Source: CAD feature listing. Evaluate the final solid. Frame: model axes, mm. Face numbers are marked on the shaded views. A direction names the side the tool comes from. Give positions to 0.01 mm unless a question says otherwise; leave off trailing zeros. Order: outer loops, then holes, each group sorted by start corner. A loop starts at its lowest first (then second) coordinate and runs counter-clockwise, first axis right, second up. Notation, with made-up numbers: M -2.5,-20.5 L 4.5,-20.5 A22 ccw 4.5,12.5 Z; hole C 2.5,0.25 d7. An arc over 180 degrees is marked long. Answer as a JSON object with one key per item and string values. Group by question number.
1. Pin query (flat end, axial travel): P1, Ø4, axis at x = -46, y = 69, coming from the -Z side; P2, Ø8, axis at x = -45, z = 15, coming from the +Y side; P3, Ø5, axis at y = 58, z = 25, coming from the +X side; P4, Ø1, axis at y = 45, z = 5, coming from the -X side. Return the tip coordinate at first contact, or that it passes through.
2. Set-up query: the marked faces 1 and 2. Return all of +Z, -Z, +X, -X, +Y, -Y with unobstructed straight access to the full face (end or side cutting, diameter ignored); none if empty.
3. Section query B-B (x = -43.75). Output: boundary loops of the cut face in (y, z), plus the area to 3 significant figures.
4. Material intervals for L1, parallel to X at y = 68, z = 29; L2, parallel to Z at x = -42.5, y = 53.5; L3, parallel to Y at x = -52.5, z = 26, sorted ascending. Write a range as [from, to].
5. Section query D-D (y = 65.5). Output: boundary loops of the cut face in (x, z).
6. Section query A-A (z = 27). Output: boundary loops of the cut face in (x, y), plus the area to 3 significant figures.
7. Section query C-C (x = -41.25). Output: boundary loops of the cut face in (y, z).
from build123d import *

# Parameters (mm, degrees)
BOSS_EXTRUDE1_DEPTH = 31.75
SKETCH19_W          = 15.860402013
SKETCH19_H          = 31.75
BOSS_EXTRUDE7_DEPTH = 2
SKETCH23_W          = 15.860402013
SKETCH23_H          = 4
BOSS_EXTRUDE8_DEPTH = 25
SKETCH24_R          = 1.27
CUT_EXTRUDE1_DEPTH  = 5


with BuildPart() as part:
    # Sketch2 → Boss-Extrude1 (new body)
    with BuildSketch(Plane.XY):
        with BuildLine():
            Line((-50.375618534, 45.609862895), (-50.351188886, 46.309436474))
            ThreePointArc((-50.351188886, 46.309436474), (-50.565618587, 46.88295476), (-51.12278195, 47.136868733))
            Line((-51.12278195, 47.136868733), (-55.780902554, 47.299533889))
            Line((-55.780902554, 47.299533889), (-47.850701548, 47.299533889))
            Line((-47.850701548, 47.299533889), (-47.850701548, 40.900752235))
            Line((-47.850701548, 40.900752235), (-48.952946324, 40.900752235))
            ThreePointArc((-48.952946324, 40.900752235), (-50.100996621, 41.129113637), (-51.074266668, 41.779431891))
            Line((-51.074266668, 41.779431891), (-53.375146928, 44.080312152))
            ThreePointArc((-53.375146928, 44.080312152), (-53.536830204, 44.931922499), (-52.803734096, 45.394471696))
            Line((-52.803734096, 45.394471696), (-50.685905631, 45.320515496))
            ThreePointArc((-50.685905631, 45.320515496), (-50.470836274, 45.400926634), (-50.375618534, 45.609862895))
        make_face()
    boss_extrude1 = extrude(amount=BOSS_EXTRUDE1_DEPTH)

    # Mirror2: Boss-Extrude1 across plane
    add(boss_extrude1.mirror(Plane(origin=(-47.850701548, 40.900752235, 31.75), x_dir=(0, 0, 1), z_dir=(-1, 0, 0))))

    # Sketch19 → Boss-Extrude7 (add)
    with BuildSketch(Plane(origin=(0, 47.299533889, 0), x_dir=(1, 0, 0), z_dir=(0, 1, 0))):
        with Locations((-47.850701548, -15.875)):
            Rectangle(SKETCH19_W, SKETCH19_H)
    extrude(amount=BOSS_EXTRUDE7_DEPTH)

    # Sketch23 → Boss-Extrude8 (add)
    with BuildSketch(Plane(origin=(0, 49.299533889, 0), x_dir=(1, 0, 0), z_dir=(0, 1, 0))):
        with Locations((-47.850701548, -29.75)):
            Rectangle(SKETCH23_W, SKETCH23_H)
    extrude(amount=BOSS_EXTRUDE8_DEPTH)

    # Sketch24 → Cut-Extrude1 (cut, through all)
    with BuildSketch(Plane(origin=(0, 0, 27.75), x_dir=(-1, 0, 0), z_dir=(0, 0, -1))):
        with Locations((47.850701548, 67.949533889)):
            Circle(SKETCH24_R)
    extrude(amount=-CUT_EXTRUDE1_DEPTH, mode=Mode.SUBTRACT)


solid = part.part
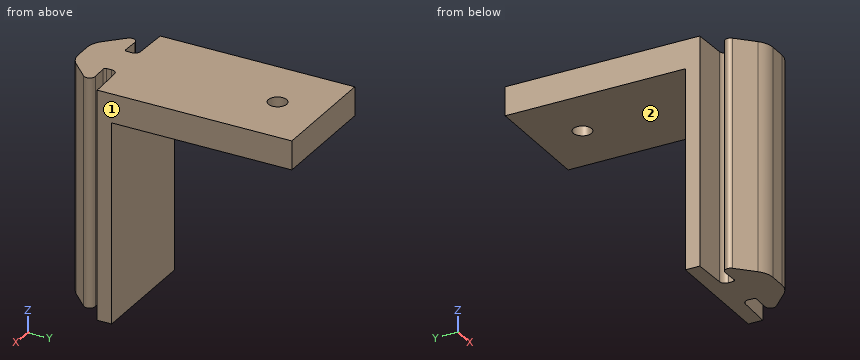
Answer sheet:
{
 "1": {"P1": "z = 27.75", "P2": "y = 49.3", "P3": "through", "P4": "x = -53.6"},
 "2": {"face 1": "+Z, -Z, +X, +Y, -Y", "face 2": "-Z, +X, -X, +Y"},
 "3": {"outline": "M 42.66,0 L 45.36,0 L 45.36,31.75 L 42.66,31.75 Z; M 47.17,0 L 49.3,0 L 49.3,27.75 L 74.3,27.75 L 74.3,31.75 L 47.17,31.75 Z", "area": "254 mm^2"},
 "4": {"L1": "[-55.78, -49.12], [-46.58, -39.92]", "L2": "[27.75, 31.75]", "L3": "[43.21, 45.38], [47.18, 49.3]"},
 "5": {"outline": "M -55.78,27.75 L -39.92,27.75 L -39.92,31.75 L -55.78,31.75 Z"},
 "6": {"outline": "M -55.78,47.3 L -51.12,47.14 A0.8 cw -50.35,46.31 L -50.38,45.61 A0.3 cw -50.69,45.32 L -52.8,45.39 A0.77 ccw -53.38,44.08 L -51.07,41.78 A3 ccw -48.95,40.9 L -46.75,40.9 A3 ccw -44.63,41.78 L -42.33,44.08 A0.77 ccw -42.9,45.39 L -45.02,45.32 A0.3 cw -45.33,45.61 L -45.35,46.31 A0.8 cw -44.58,47.14 L -39.92,47.3 L -39.92,49.3 L -55.78,49.3 Z", "area": "81.8 mm^2"},
 "7": {"outline": "M 47.25,0 L 49.3,0 L 49.3,27.75 L 74.3,27.75 L 74.3,31.75 L 47.25,31.75 Z"}
}
